Input: part model. Units: mm. Frame: model coordinates. A direction names the side the tool comes from. Round coordinates to 2 decimals unless told otherwise and drop trailing zeros. Loops run counter-clockwise (first coordinate to the right, second up) from the corner with the lowest first, then second, coordinate; pieces in that order, holes last. Notation, with made-up numbers: (3, -7) - (35, -7) arc R15 cw to (35, 3) - close; hole circle Ø7 at (69.5, 57.25). An arc over 180 degrees is marked (long way). Use CSV: the item, a comma, the result in double quotes. Start each with the question number.
1. Material intervals for probe 1 along X at (y, z) = (-17, 3); probe 2 along X at (y, z) = (21, 6.25), sorted ascending. Write a range as from..to.
2. Pull-direction query (Y, two-part tool) for faces 1 (the flat face through (-18, -60, 3)), 2 (the flat face through (18, 80, 3)), 3 (the flat face through (19.599, 15, 3)); classes: +Y half, -Y half, draft (parallel to the pull), parting line (faces both ways), or undercut.
3. Cut plane A-A (y = 44.5). Return loops of the section in (x, z), and give its area (3 significant figures).
4. Access query for faces 4 (the flat face through (19.599, -25, 3)), 5 (the flat face through (14.999, -35, 3)), 6 (the flat face through (-14.999, 45, 3)). Directions: +Z, -Z, +X, -X, +Y, -Y. A direction counts if a zero-diameter tool reaches every point of the face in a straight line with its end or side. Return the directions, or none.
5. Pin query (flat end, axial travel): P1, Ø1, axis at x = -17.5, z = 3.5, coming from the +Y side; P2, Ø1.9, axis at y = 93.5, z = 4.5, coming from the -X side; P3, Ø3, axis at x = -18, z = 2, coming from the -Y side; P4, Ø1.5, axis at x = -2, y = 56, coming from the -Z side. Return the tip coordinate at first contact, or that it passes through.
```python
from build123d import *

# Parameters (mm, degrees)
SKETCH1_W           = 29.9974
SKETCH1_H           = 200
BOSS_EXTRUDE1_DEPTH = 6.35
SKETCH2_W           = 4.6
SKETCH2_H           = 10
BOSS_EXTRUDE2_DEPTH = 6.35
LPATTERN1_COUNT     = 9
LPATTERN1_PITCH     = 20
DOGBONE01_D         = 1.5875
DOGBONE02_D         = 1.5875
LPATTERN2_COUNT     = 9
LPATTERN2_PITCH     = 20
LPATTERN4_COUNT     = 9
LPATTERN4_PITCH     = 20


with BuildPart() as part:
    # Sketch1 → Boss-Extrude1 (new body)
    with BuildSketch(Plane.XY):
        Rectangle(SKETCH1_W, SKETCH1_H)
    extrude(amount=BOSS_EXTRUDE1_DEPTH)

    # Sketch2 → Boss-Extrude2 (add)
    with BuildSketch(Plane.XY):
        with Locations((-17.2987, -85)):
            Rectangle(SKETCH2_W, SKETCH2_H)
        with Locations((17.2987, -85)):
            Rectangle(SKETCH2_W, SKETCH2_H)
    boss_extrude2 = extrude(amount=BOSS_EXTRUDE2_DEPTH)

    # LPattern1: Boss-Extrude2 ×9
    with Locations(*[(0, i * LPATTERN1_PITCH, 0) for i in range(1, LPATTERN1_COUNT)]):
        add(boss_extrude2)

    # dogBone01 (through all)
    with Locations(Plane.XY.offset(6.35)):
        with Locations((15.559966008, -90.561266008), (-15.559966008, -90.561266008)):
            dogbone01 = Hole(DOGBONE01_D / 2)

    # dogBone02 (through all)
    with Locations(Plane.XY.offset(6.35)):
        with Locations((15.559966008, -79.438733992), (-15.559966008, -79.438733992)):
            dogbone02 = Hole(DOGBONE02_D / 2)

    # LPattern2: dogBone01 ×9
    with Locations(*[(0, i * LPATTERN2_PITCH, 0) for i in range(1, LPATTERN2_COUNT)]):
        add(dogbone01, mode=Mode.SUBTRACT)

    # LPattern4: dogBone02 ×9
    with Locations(*[(0, i * LPATTERN4_PITCH, 0) for i in range(1, LPATTERN4_COUNT)]):
        add(dogbone02, mode=Mode.SUBTRACT)


solid = part.part
```
Established:
1,probe 1,"x = -15..15"
1,probe 2,"x = -14.9..14.9"
2,face 1,"undercut"
2,face 2,"+Y half"
2,face 3,"draft"
3,outline,"(-15, 0) - (15, 0) - (15, 6.35) - (-15, 6.35) - close"
3,area,"190 mm2"
4,face 4,"+Z, -Z, +X, +Y, -Y"
4,face 5,"+Z, -Z, +X"
4,face 6,"+Z, -Z, -X"
5,P1,"stops at y = 80"
5,P2,"stops at x = -15"
5,P3,"stops at y = -90"
5,P4,"stops at z = 0"
